Check sheet for the modelled part. Datum: model origin and axes. Units: mm. A direction names the side the tool comes from. Coordinates: 2 decimals unless noted, no trailing zeros. Write each loop counter-clockwise with the first axis right and the second up, starting at its lowest first coordinate (ties: lowest second). Pieces come first, ordered by that corner, then holes. Notation, with made-up numbers: M -2,41.25 L 18,41.25 A6 cw 18,48.25 Z; hole C -4,45 d6. An arc over 180 degrees is marked long. Answer as CSV lines item,"result". Start each with the question number.
1) Material ranges on L1, parallel to Z at x = 23.7, y = 35.5; L2, parallel to Z at x = 22.35, y = 27.5; L3, parallel to Y at x = 23.6, z = -6.75, recorded low to high. Write a range as [from, to].
2) Section check A-A (x = 23.8). Record the cut outline in (y, z), and give its area (3 significant figures).
3) Draft check along Y on faces 4 (the flat face through (24, 54, -8.962)), 5 (the flat face through (24, 59.6, -3)), 6 (the flat face through (24, 49.6, -7)), 7 (the cylindrical face through (25.74, -12.15, -3.27)). Enter one of: +Y half, -Y half, draft (parallel to the pull), parting line (faces both ways), or undercut.
4) Section check C-C (z = -7). Record the cut outline in (x, y).
5) Section check B-B (y = 8). Record the cut outline in (x, z), and give its area (3 significant figures).
6) Access from +Z, -Z, +X, -X, +Y, -Y to the whole of each face (thin tool, end or side, straight path). Record for faces 1 (the flat face through (22.8, 55, -7)), 2 (the flat face through (24, 51, -8.962)), 3 (the flat face through (24.8, 55, -7)).
7) Go/stop test with flat-tipped pins: pin 1 Ø4 at (y, z) = (3, -1.5) entering from -X; pin 2 Ø3.5 at (y, z) = (54.5, -7.5) entering from -X; pin 3 Ø0.5 at (x, z) = (24, -9) entering from -Y; pin 4 Ø0.5 at (x, y) = (23.5, 54.5) entering from -Z. Record where each tip stops, or that it passes through.
from build123d import *

# Parameters (mm, degrees)
PAD003_DEPTH    = 10
SKETCH021_R     = 2.75
PAD009_DEPTH    = 65
SKETCH022_R     = 1.385036
POCKET011_DEPTH = 9
SKETCH043_W     = 2.1
SKETCH043_H     = 1
POCKET021_DEPTH = 0.48
FILLET007_R     = 1


with BuildPart() as part:
    # Sketch007 → Pad003 (new body)
    with BuildSketch(Plane(origin=(-20, 60, -6), x_dir=(1, 0, 0), z_dir=(0, -1, 0))):
        with BuildLine():
            ThreePointArc((44.8, 1.638262), (43.8, 6.95), (42.8, 1.638262))
            Line((42.8, -1.461738), (42.8, 1.638262))
            Line((44.8, -1.461738), (42.8, -1.461738))
            Line((44.8, 1.638262), (44.8, -1.461738))
        make_face()
    extrude(amount=PAD003_DEPTH)

    # Sketch021 (on Face6 of Pad003) → Pad009 (join)
    with BuildSketch(Plane.XZ.offset(-50)):
        with Locations((23.8, -1.8)):
            Circle(SKETCH021_R)
    extrude(amount=PAD009_DEPTH)

    # Sketch022 → Pocket011 (cut)
    with BuildSketch(Plane.XY.offset(2)):
        with Locations((27.12612, -11.774689)):
            Circle(SKETCH022_R)
    extrude(amount=-POCKET011_DEPTH, mode=Mode.SUBTRACT)

    # Sketch043 (on Face6 of Pocket011) → Pocket021 (cut)
    with BuildSketch(Plane(origin=(0, 0, -7.461738), x_dir=(1, 0, 0), z_dir=(0, 0, -1))):
        with Locations((23.804798, -57.3)):
            Rectangle(SKETCH043_W, SKETCH043_H)
        with Locations((23.804798, -52.9)):
            Rectangle(SKETCH043_W, SKETCH043_H)
        with Locations((23.804798, -55.1)):
            Rectangle(SKETCH043_W, SKETCH043_H)
    extrude(amount=-POCKET021_DEPTH, mode=Mode.SUBTRACT)

    # Fillet007
    fillet007_edges = [part.edges().sort_by_distance(p)[0] for p in [
        (23.8, 60, -7.461738),
        (23.8, 50, -7.461738),
    ]]
    fillet(fillet007_edges, radius=FILLET007_R)


with BuildPart() as part_1:
    # Body002 placement: moved
    add(part.part.moved(Location((0, -0.4, -1.5))))


solid = part_1.part
Results found:
1,L1,"z = [-6.05, -0.55]"
1,L2,"z = [-5.64, -0.96]"
1,L3,"y = [49.6, 59.6]"
2,outline,"M -15.4,-6.05 L 49.6,-6.05 L 49.6,-7.96 A1 ccw 50.6,-8.96 L 52,-8.96 L 52,-8.48 L 53,-8.48 L 53,-8.96 L 54.2,-8.96 L 54.2,-8.48 L 55.2,-8.48 L 55.2,-8.96 L 56.4,-8.96 L 56.4,-8.48 L 57.4,-8.48 L 57.4,-8.96 L 58.6,-8.96 A1 ccw 59.6,-7.96 L 59.6,-0.55 L -15.4,-0.55 Z"
2,area,"440 mm2"
3,face 4,"draft"
3,face 5,"+Y half"
3,face 6,"-Y half"
3,face 7,"undercut"
4,outline,"M 22.8,49.6 L 24.8,49.6 L 24.8,59.6 L 22.8,59.6 Z"
5,outline,"C 23.8,-3.3 d5.5"
5,area,"23.8 mm2"
6,face 1,"-Z, -X, +Y, -Y"
6,face 2,"-Z, +X, -X, +Y, -Y"
6,face 3,"-Z, +X, +Y, -Y"
7,pin 1,"stops at x = 21.05"
7,pin 2,"stops at x = 22.55"
7,pin 3,"stops at y = 49.98"
7,pin 4,"stops at z = -8.48"
